Could you check a few things on this model? Use its own coordinates, in mm. Face numbers are marked on the shaded views. A direction names the side the tool comes from. Round coordinates to 2 decimals unless told otherwise and drop trailing zeros. Loops run counter-clockwise (first coordinate to the right, second up) from the corner with the lowest first, then second, coordinate; pieces in that order, holes last. Notation, with made-up numbers: M 33.5,1 L 83.5,1 A9 ccw 83.5,6 Z; hole C 4.5,87 d11. An arc over 180 degrees is marked long. One line per item, written item: value. Start each with the question number.
Q1. Please list where these lines run through material, in increasing order: line 1 along Z through (x, y) = (40, 7); line 2 along Y through (x, z) = (31, -47); line 3 along X through (y, z) = (4, 112).
Q2. Imagine slicing it at D-D (x = 63.5). Please give me the cut outline in (y, z), then the cut area to 3 significant figures.
Q3. I'm going to push flat-ended pins straight in: pin 1 Ø4 at (y, z) = (57, -32.5) entering from +X; pin 2 Ø12 at (y, z) = (38.5, 105.5) entering from -X; pin 3 Ø6 at (y, z) = (20, -39) entering from +X; pin 4 Ø1 at (x, z) = (49, -55.5) entering from +Y. Where does each tip first touch, or does it pass through?
Q4. Imagine slicing it at A-A (x = 40). Please give me the cut outline in (y, z), then the cut area to 3 significant figures.
Q5. Which directions (+Z, -Z, +X, -X, +Y, -Y) give clear straight access to the entire face, cutting with the end or side of a thin tool? Please do the marked faces 1 and 2.
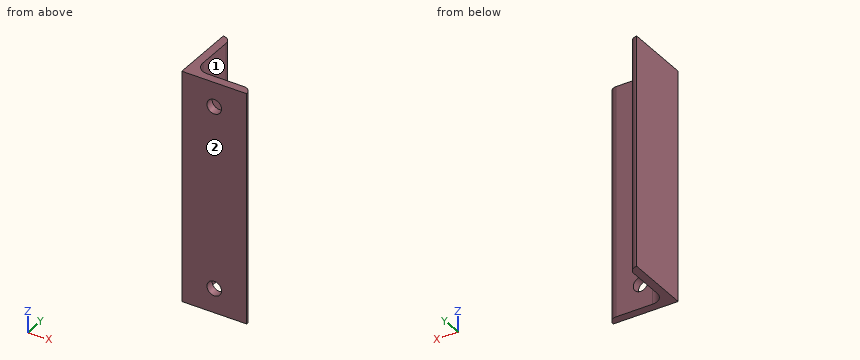
Autodesk Fusion 360 part; units mm, degrees
sketch "Sketch1" plane through (0, 0, 0) normal (0, 0, 1) x (1, 0, 0)
  line L0 (0, 0) -> (80, 0)
  line L1 (0, 0) -> (0, 80)
  line L2 (0, 80) -> (10, 80)
  line L3 (80, 0) -> (80, 10)
  line L4 (10, 80) -> (10, 10)
  line L5 (10, 10) -> (80, 10)
  dimension "d1" = 80
  dimension "d2" = 80
  dimension "d3" = 10
  dimension "d4" = 10
extrude "Extrude1" add sketch "Sketch1" along normal mid plane 285
fillet "Fillet1" radius 10 2 edges at (80, 10, 0) (10, 80, 0)
fillet "Fillet2" radius 15 1 edges at (10, 10, 0)
sketch "Sketch2" plane through (0, 0, 0) normal (0, -1, 0) x (1, 0, 0)
  line L0 (80, -142.5) -> (80, 142.5)
  line L1 (80, 142.5) -> (0, 142.5)
  line L2 (0, 142.5) -> (0, -142.5)
  line L3 (0, -142.5) -> (80, -142.5)
  circle A0 centre (40, 112.5) radius 9
  line L4 (25, -142.5) -> (70, -142.5)
  line L5 (40, 142.5) -> (40, -142.5) construction
  line L6 (40, 142.5) -> (40, 112.5) construction
  line L7 (0, 0) -> (80, 0) construction
  circle A1 centre (40, -112.5) radius 9
  dimension "d9" = 18
  dimension "d10" = 30
extrude "Extrude2" cut sketch "Sketch2" against normal through all contours A0 | A1
Report:
1. line 1: z = -142.5 to -121.5, -103.5 to 103.5, 121.5 to 142.5
1. line 2: y = 0 to 10
1. line 3: x = 0 to 31.01, 48.99 to 79.17
2. outline: M 0,-142.5 L 10,-142.5 L 10,142.5 L 0,142.5 Z
2. area: 2,850 mm²
3. pin 1: stops at x = 10
3. pin 2: stops at x = 0
3. pin 3: stops at x = 12.31
3. pin 4: stops at y = 10
4. outline: M 0,-142.5 L 10,-142.5 L 10,-121.5 L 0,-121.5 Z; M 0,-103.5 L 10,-103.5 L 10,103.5 L 0,103.5 Z; M 0,121.5 L 10,121.5 L 10,142.5 L 0,142.5 Z
4. area: 2,490 mm²
5. face 1: +Z, -Z, +X, +Y
5. face 2: +Z, -Z, +X, -X, -Y
